Model file for the job. Use its own axes, mm. A direction names the side the tool comes from. Coordinates: 2 decimals unless noted, no trailing zeros. Order: outer loops, then holes, each group sorted by start corner. A loop starts at its lowest first (then second) coordinate and runs counter-clockwise, first axis right, second up. Notation, with made-up numbers: M -27,-12.75 L 23,-12.75 A21 cw 23,7.25 Z; hole C -39,79 d6. An arc over 180 degrees is marked long. Return JSON: item names as keys, results as strings.
```python
from build123d import *

# Parameters (mm, degrees)
F0_R     = 2.5
F1_DEPTH = 3
F2_R     = 4


with BuildPart() as f1:
    # F0 (on Top) → F1 (new body)
    with BuildSketch(Plane.XY):
        with BuildLine():
            Line((-37.006066629, 43.3700063947), (-63.2541444994, 43.3700063947))
            Line((-63.2541444994, 43.3700063947), (-63.2541444994, 5.3700063947))
            Line((-63.2541444994, 5.3700063947), (-37.006066629, 5.3700063947))
            ThreePointArc((-37.006066629, 5.3700063947), (-54.1541444994, 24.3700063947), (-37.006066629, 43.3700063947))
        make_face()
        with BuildLine():
            Line((-6.8541444994, 43.3700063947), (-33.1022223698, 43.3700063947))
            ThreePointArc((-33.1022223698, 43.3700063947), (-20.8750804845, 37.1670429135), (-15.9541444994, 24.3700063947))
            ThreePointArc((-15.9541444994, 24.3700063947), (-20.8750804845, 11.572969876), (-33.1022223698, 5.3700063947))
            Line((-33.1022223698, 5.3700063947), (-6.8541444994, 5.3700063947))
            Line((-6.8541444994, 5.3700063947), (-6.8541444994, 43.3700063947))
        make_face()
        with BuildLine():
            ThreePointArc((-74.5541444994, 32.3700063947), (-68.8972902499, 30.0268606442), (-66.5541444994, 24.3700063947))
            ThreePointArc((-66.5541444994, 24.3700063947), (-68.8972902499, 18.7131521453), (-74.5541444994, 16.3700063947))
            Line((-74.5541444994, 16.3700063947), (-84.4726338983, 16.3700063947))
            Line((-84.4726338983, 16.3700063947), (-84.4726338983, 5.3700063947))
            Line((-84.4726338983, 5.3700063947), (-63.2541444994, 5.3700063947))
            Line((-63.2541444994, 5.3700063947), (-63.2541444994, 43.3700063947))
            Line((-63.2541444994, 43.3700063947), (-84.4726338983, 43.3700063947))
            Line((-84.4726338983, 43.3700063947), (-84.4726338983, 32.3700063947))
            Line((-84.4726338983, 32.3700063947), (-74.5541444994, 32.3700063947))
        make_face()
        with Locations((-74.5541444994, 10.3700063947)):
            Circle(F0_R, mode=Mode.SUBTRACT)
        with Locations((-74.5541444994, 38.3700063947)):
            Circle(F0_R, mode=Mode.SUBTRACT)
        with BuildLine():
            Line((14.3643448995, 43.3700063947), (-6.8541444994, 43.3700063947))
            Line((-6.8541444994, 43.3700063947), (-6.8541444994, 5.3700063947))
            Line((-6.8541444994, 5.3700063947), (14.3643448995, 5.3700063947))
            Line((14.3643448995, 5.3700063947), (14.3643448995, 16.3700063947))
            Line((14.3643448995, 16.3700063947), (4.4458555006, 16.3700063947))
            ThreePointArc((4.4458555006, 16.3700063947), (-3.5541444994, 24.3700063947), (4.4458555006, 32.3700063947))
            Line((4.4458555006, 32.3700063947), (14.3643448995, 32.3700063947))
            Line((14.3643448995, 32.3700063947), (14.3643448995, 43.3700063947))
        make_face()
        with Locations((4.4458555006, 10.3700063947)):
            Circle(F0_R, mode=Mode.SUBTRACT)
        with Locations((4.4458555006, 38.3700063947)):
            Circle(F0_R, mode=Mode.SUBTRACT)
        with BuildLine():
            Line((-37.006066629, 5.3700063947), (-63.2541444994, 5.3700063947))
            Line((-63.2541444994, 5.3700063947), (-63.2541444994, -3.8299936053))
            Line((-63.2541444994, -3.8299936053), (-6.8541444994, -3.8299936053))
            Line((-6.8541444994, -3.8299936053), (-6.8541444994, 5.3700063947))
            Line((-6.8541444994, 5.3700063947), (-33.1022223698, 5.3700063947))
            ThreePointArc((-33.1022223698, 5.3700063947), (-35.0541444994, 5.2700063947), (-37.006066629, 5.3700063947))
        make_face()
        with Locations((-58.6241444994, 0.8000063947)):
            Circle(F0_R, mode=Mode.SUBTRACT)
        with Locations((-11.4841444994, 0.8000063947)):
            Circle(F0_R, mode=Mode.SUBTRACT)
        with BuildLine():
            Line((-63.2541444994, 52.5700063947), (-63.2541444994, 43.3700063947))
            Line((-63.2541444994, 43.3700063947), (-37.006066629, 43.3700063947))
            ThreePointArc((-37.006066629, 43.3700063947), (-36.8681827001, 43.3836663635), (-36.7302033051, 43.3963257151))
            ThreePointArc((-36.7302033051, 43.3963257151), (-35.0541444994, 43.4700063947), (-33.3780856936, 43.3963257151))
            ThreePointArc((-33.3780856936, 43.3963257151), (-33.2401062987, 43.3836663635), (-33.1022223698, 43.3700063947))
            Line((-33.1022223698, 43.3700063947), (-6.8541444994, 43.3700063947))
            Line((-6.8541444994, 43.3700063947), (-6.8541444994, 52.5700063947))
            Line((-6.8541444994, 52.5700063947), (-63.2541444994, 52.5700063947))
        make_face()
        with Locations((-58.6241444994, 47.9400063947)):
            Circle(F0_R, mode=Mode.SUBTRACT)
        with Locations((-11.4841444994, 47.9400063947)):
            Circle(F0_R, mode=Mode.SUBTRACT)
    extrude(amount=F1_DEPTH)

    # F2
    f2_edges = [f1.edges().sort_by_distance(p)[0] for p in [
        (-6.854144, 52.570006, 1.5),
        (14.364345, 43.370006, 1.5),
        (14.364345, 5.370006, 1.5),
        (-6.854144, -3.829994, 1.5),
        (-63.254144, 52.570006, 1.5),
        (-84.472634, 43.370006, 1.5),
        (-84.472634, 16.370006, 1.5),
        (-84.472634, 32.370006, 1.5),
        (-84.472634, 5.370006, 1.5),
        (-63.254144, -3.829994, 1.5),
        (14.364345, 32.370006, 1.5),
        (14.364345, 16.370006, 1.5),
        (-6.854144, 43.370006, 1.5),
        (-6.854144, 5.370006, 1.5),
        (-63.254144, 5.370006, 1.5),
        (-63.254144, 43.370006, 1.5),
    ]]
    fillet(f2_edges, radius=F2_R)


solid = f1.part
```
Item 1: Saw through at C-C (z = 1.2). Count the separate pieces of the cut face and the enclosed holes in it, and give its area (3 significant figures).
Check result:
{"separate pieces": "1", "enclosed holes": "9", "area": "2,940 mm2"}
Item 2: Pull direction X, two halves, no side cores. Call faces 1 (the cylindrical face through (-61.12, 48.05, 1.48)), 2 (the flat face through (4, 43.37, 1)), 3 (the cylindrical face through (13.16, 42.23, 1.52)): +X half, -X half, draft (parallel to the pull), parting line (faces both ways), or undercut.
Check result:
{"face 1": "undercut", "face 2": "draft", "face 3": "+X half"}
Item 3: Saw through at A-A (x = -47.5). Write the cut outline in (y, z), and give its area (3 significant figures).
Check result:
{"outline": "M -3.83,0 L 9.88,0 L 9.88,3 L -3.83,3 Z; M 38.86,0 L 52.57,0 L 52.57,3 L 38.86,3 Z", "area": "82.3 mm2"}
Item 4: 3-axis set-ups, long thin cutter, end or side, ignore diameter. For faces 4 (the flat face through (4, 5.37, 1)), 5 (the cylindrical face through (13.16, 15.23, 1.52)), 6 (the cylindrical face through (-83.3, 15.2, 1.5)), 7 (the flat face through (-74, 5.37, 1)): which of +Z, -Z, +X, -X, +Y, -Y reach the whole face in a straight line?
Check result:
{"face 4": "+Z, -Z, +X, -Y", "face 5": "+Z, -Z, +X", "face 6": "+Z, -Z, -X", "face 7": "+Z, -Z, -X, -Y"}
Item 5: Drop flat-ended pins along their axis: pin 1 Ø1.3 at (y, z) = (0.5, 2) entering from -X; pin 2 Ø0.6 at (y, z) = (48, 1.5) entering from +X. Give the stop position or say it passes through.
Check result:
{"pin 1": "stops at x = -63.25", "pin 2": "stops at x = -6.85"}
Item 6: Wall check: line 1 (Y direction, x = -74.5, z = 2.6); line 2 (Y direction, x = -12, z = 0.8); line 3 (X direction, y = 3, z = 0.1). Give the ranges that are in metal, low to high.
Check result:
{"line 1": "y = 5.37 to 7.87, 12.87 to 16.37, 32.37 to 35.87, 40.87 to 43.37", "line 2": "y = -3.83 to -1.65, 3.25 to 45.49, 50.39 to 52.57", "line 3": "x = -63.6 to -59.81, -57.44 to -12.67, -10.3 to -6.51"}
Item 7: Saw through at B-B (y = 14.5). Write the cut outline in (x, z).
Check result:
{"outline": "M -83.86,0 L -51.41,0 L -51.41,3 L -83.86,3 Z; M -18.7,0 L 13.75,0 L 13.75,3 L -18.7,3 Z"}
